from build123d import *

# Parameters (mm, degrees)
SKETCH1_R                                        = 12.7
BASE_EXTRUDE_DEPTH                               = 16.5
CBORE_FOR_1_4_SOCKET_HEAD_CAP_SCREW1_D           = 6.5278
CBORE_FOR_1_4_SOCKET_HEAD_CAP_SCREW1_CBORE_D     = 11.1125
CBORE_FOR_1_4_SOCKET_HEAD_CAP_SCREW1_CBORE_DEPTH = 6.35
SKETCH4_W                                        = 26.942464066
SKETCH4_H                                        = 0.25
VENT_GROOVE_FRONT_DEPTH                          = 0.25
SKETCH5_W                                        = 27.489916166
SKETCH5_H                                        = 0.25
VENT_GROOVE_BACK_DEPTH                           = 0.25


with BuildPart() as part:
    # Sketch1 → Base-Extrude (new body)
    with BuildSketch(Plane.XY):
        Circle(SKETCH1_R)
    extrude(amount=BASE_EXTRUDE_DEPTH)

    # CBORE for 1/4 Socket Head Cap Screw1 (through all)
    with Locations(Plane(origin=(7.46029001, -0.504629161, 16.5), x_dir=(1, 0, 0), z_dir=(0, 0, 1))):
        with Locations((-7.46029001, 0.504629161)):
            CounterBoreHole(CBORE_FOR_1_4_SOCKET_HEAD_CAP_SCREW1_D / 2, CBORE_FOR_1_4_SOCKET_HEAD_CAP_SCREW1_CBORE_D / 2, CBORE_FOR_1_4_SOCKET_HEAD_CAP_SCREW1_CBORE_DEPTH)

    # Sketch4 → Vent Groove Front (cut)
    with BuildSketch(Plane.XY.offset(16.5)):
        with Locations((0.293277911, 0)):
            Rectangle(SKETCH4_W, SKETCH4_H)
    extrude(amount=-VENT_GROOVE_FRONT_DEPTH, mode=Mode.SUBTRACT)

    # Sketch5 → Vent Groove Back (cut)
    with BuildSketch(Plane(origin=(0, 0, 0), x_dir=(-1, 0, 0), z_dir=(0, 0, -1))):
        with Locations((0.254174189, 0)):
            Rectangle(SKETCH5_W, SKETCH5_H)
    extrude(amount=-VENT_GROOVE_BACK_DEPTH, mode=Mode.SUBTRACT)


solid = part.part
Here's how the part is built. I have some questions about the finished solid (model axes, mm). A direction names the side the tool comes from. Coordinates: 2 decimals unless noted, no trailing zeros. Order: outer loops, then holes, each group sorted by start corner. A loop starts at its lowest first (then second) coordinate and runs counter-clockwise, first axis right, second up. Notation, with made-up numbers: (56.25, -26.75) - (82.25, -26.75) arc R29 ccw to (82.25, 7.25) - close; hole circle Ø5 at (68.5, 10.25). An arc over 180 degrees is marked (long way). Use CSV: the item, a comma, the result in double quotes. Start each with the question number.
1. Suppose I cut it at A-A on x = 0. List the corners of the cut face in (y, z) for me, then the cut area to 3 significant figures.
2. I'm going to push a flat-ended pin straight in: pin 1 (9 mm diameter, centred on x = -2.5, y = 0.5, fed in from +Z). Where does the tip first touch, or does it pass through?
3. If we mould it in two halves opening along Y, with no side actions, what happens to faces 1 (the face through (-2.75, -12.4, 8.13)), 2 (the face through (0, -4, 10.15)), 3 (the face through (0, -6, 16.5))? For each: +Y half, -Y half, draft (parallel to the pull), parting line (faces both ways), or undercut.
4. Please list where these lines run through material, in increasing order: line 1 (X direction, y = 0, z = 4.5); line 2 (Y direction, x = 0, z = 14.75). Write a range as from..to.
5. Suppose I cut it at C-C on z = 8. List the corners of the cut face in (x, y) for me.
6. For faces 4 (the face through (0, -6, 0)), 5 (the face through (5.3, 1.67, 13.37)), which set-ups out of +Z, -Z, +X, -X, +Y, -Y let a thin tool reach every point of the face, with its end or its side?
7. Suppose I cut it at D-D on x = -4.25. List the corners of the cut face in (y, z) for me (3 decimals), then the cut area to 3 significant figures.
8. Suppose I cut it at B-B on y = 2.5. List the corners of the cut face in (x, z) for me, then the cut area to 3 significant figures.
Output:
1,outline,"(-12.7, 0) - (-3.26, 0) - (-3.26, 10.15) - (-5.56, 10.15) - (-5.56, 16.5) - (-12.7, 16.5) - close; (3.26, 0) - (12.7, 0) - (12.7, 16.5) - (5.56, 16.5) - (5.56, 10.15) - (3.26, 10.15) - close"
1,area,"282 mm2"
2,pin 1,"stops at z = 16.5"
3,face 1,"parting line"
3,face 2,"undercut"
3,face 3,"draft"
4,line 1,"x = -12.7..-3.26, 3.26..12.7"
4,line 2,"y = -12.7..-5.56, 5.56..12.7"
5,outline,"circle Ø25.4 at (0, 0); hole circle Ø6.53 at (0, 0)"
6,face 4,"-Z, +X, -X, +Y, -Y"
6,face 5,"+Z"
7,outline,"(-11.968, 0) - (-0.125, 0) - (-0.125, 0.25) - (0.125, 0.25) - (0.125, 0) - (11.968, 0) - (11.968, 16.5) - (3.579, 16.5) - (3.579, 10.15) - (-3.579, 10.15) - (-3.579, 16.5) - (-11.968, 16.5) - close"
7,area,"349 mm2"
8,outline,"(-12.45, 0) - (-2.1, 0) - (-2.1, 10.15) - (-4.96, 10.15) - (-4.96, 16.5) - (-12.45, 16.5) - close; (2.1, 0) - (12.45, 0) - (12.45, 16.5) - (4.96, 16.5) - (4.96, 10.15) - (2.1, 10.15) - close"
8,area,"305 mm2"
